```python
from build123d import *

# Parameters (mm, degrees)
SKETCH1_W           = 3.175
SKETCH1_H           = 9.525
SKETCH1_W_2         = 8.308704394
SKETCH1_H_2         = 2.54
BOSS_EXTRUDE1_DEPTH = 7
BOSS_EXTRUDE2_DEPTH = 1.5875


with BuildPart() as part:
    # Sketch1 → Boss-Extrude1 (new body)
    with BuildSketch(Plane.XY):
        with BuildLine():
            ThreePointArc((0, -3.4), (-3.343276836, -0.618465844), (-1.216295606, 3.175))
            Line((-1.216295606, 3.175), (-6.35, 3.175))
            Line((-6.35, 3.175), (-6.35, -6.35))
            Line((-6.35, -6.35), (0, -6.35))
            Line((0, -6.35), (0, -3.4))
        make_face()
        with Locations((-7.9375, -1.5875)):
            Rectangle(SKETCH1_W, SKETCH1_H)
        with Locations((-5.370647803, 4.445)):
            Rectangle(SKETCH1_W_2, SKETCH1_H_2)
    extrude(amount=BOSS_EXTRUDE1_DEPTH)

    # Sketch2 → Boss-Extrude2 (add)
    with BuildSketch(Plane.XY.offset(7)):
        with BuildLine():
            Line((-1.216295606, 3.175), (-1.216295606, 5.715))
            Line((-1.216295606, 5.715), (-9.525, 5.715))
            Line((-9.525, 5.715), (-9.525, -6.35))
            Line((-9.525, -6.35), (-1.216295606, -6.35))
            Line((-1.216295606, -6.35), (-1.216295606, -3.175))
            ThreePointArc((-1.216295606, -3.175), (-3.4, 0), (-1.216295606, 3.175))
        make_face()
        with BuildLine():
            Line((-1.216295606, 2.851425082), (-1.216295606, 3.175))
            ThreePointArc((-1.216295606, 3.175), (-3.4, 0), (-1.216295606, -3.175))
            Line((-1.216295606, -3.175), (-1.216295606, -2.851425082))
            ThreePointArc((-1.216295606, -2.851425082), (-3.1, 0), (-1.216295606, 2.851425082))
        make_face()
        with BuildLine():
            Line((-1.216295606, -2.851425082), (-1.216295606, -3.175))
            ThreePointArc((-1.216295606, -3.175), (-0.618465844, -3.343276836), (0, -3.4))
            Line((0, -3.4), (0, -3.1))
            ThreePointArc((0, -3.1), (-0.620718231, -3.037220584), (-1.216295606, -2.851425082))
        make_face()
        with BuildLine():
            ThreePointArc((0, -3.4), (-0.618465844, -3.343276836), (-1.216295606, -3.175))
            Line((-1.216295606, -3.175), (-1.216295606, -6.35))
            Line((-1.216295606, -6.35), (0, -6.35))
            Line((0, -6.35), (0, -3.4))
        make_face()
        with BuildLine():
            Line((0, 5.715), (-1.216295606, 5.715))
            Line((-1.216295606, 5.715), (-1.216295606, 3.175))
            Line((-1.216295606, 3.175), (-1.216295606, 2.851425082))
            ThreePointArc((-1.216295606, 2.851425082), (-0.620718231, 3.037220584), (0, 3.1))
            Line((0, 3.1), (0, 5.715))
        make_face()
    boss_extrude2 = extrude(amount=BOSS_EXTRUDE2_DEPTH)

    # Mirror1: Boss-Extrude2 across plane
    add(boss_extrude2.mirror(Plane.XY.offset(3.5)))


solid = part.part
```
The listing builds one solid part. Answer for the finished solid, in the listing's coordinates (mm). Give positions to 0.01 mm unless a question says otherwise; leave off trailing zeros. Write each loop counter-clockwise with the first axis right and the second up, starting at its lowest first coordinate (ties: lowest second). Pieces come first, ordered by that corner, then holes. Notation, with made-up numbers: (34, 33.5) -> (85, 33.5) arc R14 ccw to (85, 50.5) -> close; hole circle Ø5 at (56.5, 2). An arc over 180 degrees is marked (long way). Write item = value, one per line. Start each with the question number.
1) Straight lines are drawn through the part: line 1 along Z through (x, y) = (-3.25, 0.25); line 2 along X through (y, z) = (5, 5.5) (3 decimals); line 3 along Y through (x, z) = (-1.25, 1.5) (3 decimals). For each, find the intervals that lie inside material, in ascending order.
2) The part is cut by section A-A, the plane y = 4.75. Determine the outline of the cut face in (x, z) (1 decimal).
3) Determine the mould class of faces 1 (the face through (-1.216, 4, 3)), 2 (the face through (-3.33, -0.68, 3.45)), 3 (the face through (-5, -6.35, 4)) for opening direction Y: +Y half, -Y half, draft (parallel to the pull), parting line (faces both ways), or undercut.
4) The part is cut by section D-D, the plane z = 5.5. Determine the outline of the cut face in (x, y) (3 decimals).
5) The part is cut by section C-C, the plane z = 7.5. Determine the outline of the cut face in (x, y) (3 decimals), and give its area (3 significant figures).
6) This flat-tipped pin is pushed along its axis until it touches: pin 1 (3 mm diameter, centred on y = 4, z = 3, fed in from +X). Where does it stop, or does it pass through?
Solutions:
q1.line_1 = -1.59 to 0, 7 to 8.59
q1.line_2 = -9.525 to -1.216
q1.line_3 = -6.35 to -3.162, 3.162 to 5.715
q2.outline = (-9.5, -1.6) -> (0, -1.6) -> (0, 0) -> (-1.2, 0) -> (-1.2, 7) -> (0, 7) -> (0, 8.6) -> (-9.5, 8.6) -> close
q3.face_1 = draft
q3.face_2 = undercut
q3.face_3 = -Y half
q4.outline = (-9.525, -6.35) -> (0, -6.35) -> (0, -3.4) arc R3.4 cw to (-1.216, 3.175) -> (-1.216, 5.715) -> (-9.525, 5.715) -> close
q5.outline = (-9.525, -6.35) -> (0, -6.35) -> (0, -3.1) arc R3.1 cw to (0, 3.1) -> (0, 5.715) -> (-9.525, 5.715) -> close
q5.area = 99.8 mm²
q6.pin_1 = -1.22
